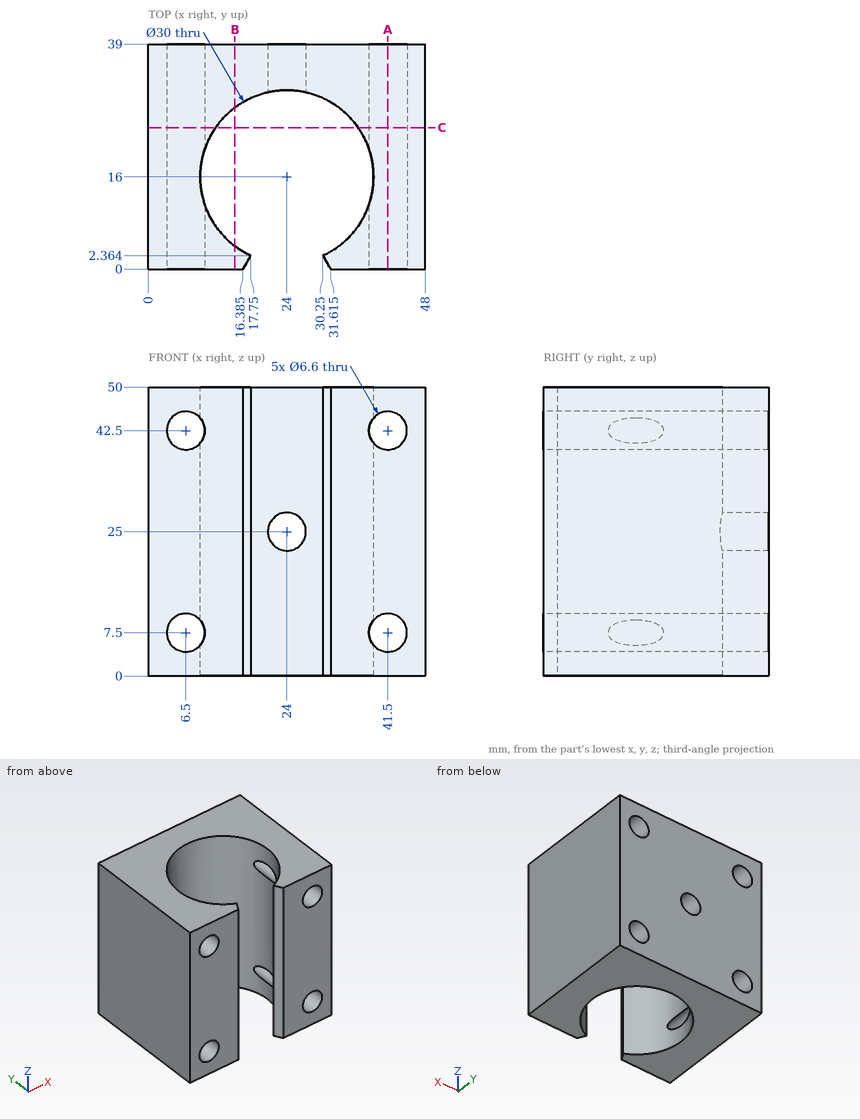
Verification items for this drawing (mm, ordinates from the low corner). Give positions to 0.01 mm unless a question says otherwise; leave off trailing zeros. Loops run counter-clockwise (first coordinate to the right, second up) from the corner with the lowest first, then second, coordinate; pieces in that order, holes last.
(1) Thickness scan on L1, parallel to Z at x = 41.5, y = 16; L2, parallel to X at y = 2, z = 6; L3, parallel to X at y = 28, z = 8. Record the ranges inside material, lowest first.
From the geometry:
L1: z = 0 to 4.2, 10.8 to 39.2, 45.8 to 50
L2: x = 0 to 3.56, 9.44 to 17.54, 30.46 to 38.56, 44.44 to 48
L3: x = 0 to 3.24, 9.76 to 15, 33 to 38.24, 44.76 to 48
(2) Section check A-A on x = 41.5. Record the cut outline in (y, z), then the cut area to 3 significant figures.
From the geometry:
outline: (0, 0) - (39, 0) - (39, 4.2) - (0, 4.2) - close; (0, 10.8) - (39, 10.8) - (39, 39.2) - (0, 39.2) - close; (0, 45.8) - (39, 45.8) - (39, 50) - (0, 50) - close
area: 1,440 mm2
(3) Section check C-C on y = 24.5. Record the cut outline in (x, z).
From the geometry:
outline: (0, 0) - (11.64, 0) - (11.64, 50) - (0, 50) - close; (36.36, 0) - (48, 0) - (48, 50) - (36.36, 50) - close; hole circle Ø6.6 at (6.5, 7.5); hole circle Ø6.6 at (6.5, 42.5); hole circle Ø6.6 at (41.5, 7.5); hole circle Ø6.6 at (41.5, 42.5)
(4) Section check B-B on x = 15. Record the cut outline in (y, z), then the cut area to 3 significant figures.
From the geometry:
outline: (0, 0) - (4, 0) - (4, 50) - (0, 50) - close; (28, 0) - (39, 0) - (39, 50) - (28, 50) - close
area: 750 mm2
